Design review of the part built by this model. Coordinates are the model's own, in mm. A direction names the side the tool comes from. Round coordinates to 2 decimals unless told otherwise and drop trailing zeros. Order: outer loops, then holes, each group sorted by start corner. A loop starts at its lowest first (then second) coordinate and runs counter-clockwise, first axis right, second up. Notation, with made-up numbers: M 50,59 L 96,59 A12 ccw 96,67 Z; hole C 8.5,50.25 d4. An arc over 180 degrees is marked long. Write each question's results on one line, items separated by ' | '. Start each with the question number.
Item 1: Take a section at D-D, the plane y = 6. Write out the cut boundary in (x, z), plus the area to 3 significant figures.
Item 2: Clearance check with flat-ended pins moving along their axes: pin 1 (1.5 mm diameter, centred on x = 3, y = 7.5, fed in from +Z); pin 2 (3 mm diameter, centred on x = 0, z = 0, fed in from +Y); pin 3 (4 mm diameter, centred on x = 4.5, y = 1.5, fed in from -Z). State where each tip first meets the part, or that it passes through.
Item 3: The part is to be moulded in two halves that separate along Z. For faces 1 (the conical face through (-0.28, 2.234, -0.062)), 2 (the flat face through (3, 7.185, -5)), 3 (the cylindrical face through (-1.19, 7.75, -5.37)), say which applies: +Z half, -Z half, draft (parallel to the pull), parting line (faces both ways), or undercut.
Item 4: Take a section at A-A, the plane y = 7.75. Write out the cut boundary in (x, z).
Item 5: Wall thickness on line 1 (Y direction, x = -4.5, z = 3.5); line 2 (Z direction, x = 0, y = 7); line 3 (Z direction, x = 0, y = 7.25): over which ranges is each line inside the solid? List them lowest first. Write a range as [from, to].
Item 6: Take a section at B-B, the plane x = -3.5. Write out the cut boundary in (y, z), plus the area to 3 significant figures.
Item 7: Machinability: for faces 4 (the cylindrical face through (1.115, 6.997, 1.216)), 5 (the cylindrical face through (-6, 6, 0)), 6 (the cylindrical face through (-1.19, 3.32, -5.37)), which of the approach directions +Z, -Z, +X, -X, +Y, -Y give a long, thin tool a straight path to every point of the face, cutting with its end or side? Answer none if there is none.
Item 8: Take a section at C-C, the plane y = 1.75. Write out the cut boundary in (x, z), plus the area to 3 significant figures.
```python
from build123d import *

# Parameters (mm, degrees)
M4X0_7_TAPPED_HOLE1_D     = 3.3
M4X0_7_TAPPED_HOLE1_DEPTH = 8
M4X0_7_TAPPED_HOLE1_TIP   = 0.991420021


with BuildPart() as part:
    # Sketch2 → Revolve1 (revolve)
    with BuildSketch(Plane.XY):
        Polygon((0, 0), (6, 0), (6, 2.762622939), (5.5, 2.762622939), (5.5, 3.867672115), (6, 3.867672115), (6, 7.185259401), (5.5, 7.185259401), (5.5, 8.290308577), (6, 8.290308577), (6, 11.052931516), (0, 11.052931516), align=None)
    revolve(axis=Axis((0, 48.827905014, 0), (0, -1, 0)))

    # M4x0.7 Tapped Hole1
    with Locations(Plane.ZX.offset(11.052931516)):
        with Locations((0, 0)):
            Hole(M4X0_7_TAPPED_HOLE1_D / 2, depth=M4X0_7_TAPPED_HOLE1_DEPTH)
            with Locations((0, 0, -(M4X0_7_TAPPED_HOLE1_DEPTH + M4X0_7_TAPPED_HOLE1_TIP / 2))):  # 118° drill point
                Cone(0, M4X0_7_TAPPED_HOLE1_D / 2, M4X0_7_TAPPED_HOLE1_TIP, mode=Mode.SUBTRACT)


solid = part.part
```
Results list:
1) outline: C 0,0 d12; hole C 0,0 d3.3 | area: 105 mm²
2) pin 1: z = 5.53 | pin 2: y = 2.96 | pin 3: z = -5.45
3) face 1: undercut | face 2: draft | face 3: parting line
4) outline: C 0,0 d11; hole C 0,0 d3.3
5) line 1: [0, 2.76], [3.87, 7.19], [8.29, 11.05] | line 2: [-6, -1.65], [1.65, 6] | line 3: [-5.5, -1.65], [1.65, 5.5]
6) outline: M 0,-4.87 L 2.76,-4.87 L 2.76,-4.24 L 3.87,-4.24 L 3.87,-4.87 L 7.19,-4.87 L 7.19,-4.24 L 8.29,-4.24 L 8.29,-4.87 L 11.05,-4.87 L 11.05,4.87 L 8.29,4.87 L 8.29,4.24 L 7.19,4.24 L 7.19,4.87 L 3.87,4.87 L 3.87,4.24 L 2.76,4.24 L 2.76,4.87 L 0,4.87 Z | area: 105 mm²
7) face 4: +Y | face 5: +Y, -Y | face 6: none
8) outline: C 0,0 d12 | area: 113 mm²
